Geometry: see drawing. Coordinates: mm, zero at the bounding-box minimum. Coordinates: 2 decimals unless noted, no trailing zeros. Loops run counter-clockwise (first coordinate to the right, second up) from the corner with the lowest first, then second, coordinate; pieces in that order, holes last. Notation, with made-up numbers: (-11, -26) -> (-7, -26) arc R27 ccw to (-7, -4) -> close; hole circle Ø5 at (43.5, -28). An arc over 180 degrees is marked (long way). Answer as a JSON object with one key per item and string values.
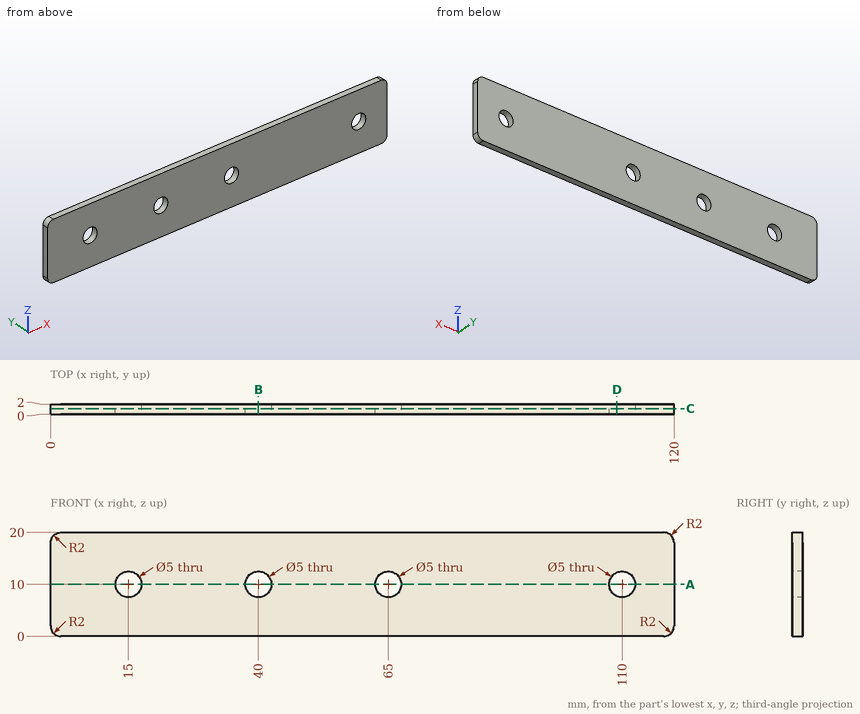
1. Section query C-C (y = 1.1). Return loops of the section in (x, z), plus the area to 3 significant figures.
Reply:
{"outline": "(0, 2) arc R2 ccw to (2, 0) -> (118, 0) arc R2 ccw to (120, 2) -> (120, 18) arc R2 ccw to (118, 20) -> (2, 20) arc R2 ccw to (0, 18) -> close; hole circle Ø5 at (15, 10); hole circle Ø5 at (40, 10); hole circle Ø5 at (65, 10); hole circle Ø5 at (110, 10)", "area": "2,320 mm2"}
2. Pin query (flat end, axial travel): P1, Ø1, axis at x = 67, z = 17.5, coming from the -Y side. Return the tip coordinate at first contact, or that it passes through.
Reply:
{"P1": "stops at y = 0"}
3. Section query A-A (z = 10). Return loops of the section in (x, y), plus the area to 3 significant figures.
Reply:
{"outline": "(0, 0) -> (12.5, 0) -> (12.5, 2) -> (0, 2) -> close; (17.5, 0) -> (37.5, 0) -> (37.5, 2) -> (17.5, 2) -> close; (42.5, 0) -> (62.5, 0) -> (62.5, 2) -> (42.5, 2) -> close; (67.5, 0) -> (107.5, 0) -> (107.5, 2) -> (67.5, 2) -> close; (112.5, 0) -> (120, 0) -> (120, 2) -> (112.5, 2) -> close", "area": "200 mm2"}
4. Section query D-D (x = 109). Return loops of the section in (y, z), plus the area to 3 significant figures.
Reply:
{"outline": "(0, 0) -> (2, 0) -> (2, 7.71) -> (0, 7.71) -> close; (0, 12.29) -> (2, 12.29) -> (2, 20) -> (0, 20) -> close", "area": "30.8 mm2"}
5. Section query B-B (x = 40). Return loops of the section in (y, z).
Reply:
{"outline": "(0, 0) -> (2, 0) -> (2, 7.5) -> (0, 7.5) -> close; (0, 12.5) -> (2, 12.5) -> (2, 20) -> (0, 20) -> close"}
6. Line query: line 1 along Z through (x, y) = (15, 1.1); line 2 along X through (y, z) = (1.3, 8.75); line 3 along X through (y, z) = (0.25, 1.5). Output: solid intervals per line, ascending.
Reply:
{"line 1": "z = 0 to 7.5, 12.5 to 20", "line 2": "x = 0 to 12.83, 17.17 to 37.83, 42.17 to 62.83, 67.17 to 107.83, 112.17 to 120", "line 3": "x = 0.06 to 119.94"}
